Autodesk Inventor part; units mm, degrees
ref_plane "YZ Plane" through (0, 0, 0) normal (1, 0, 0) x (0, 1, 0)
ref_plane "XZ Plane" through (0, 0, 0) normal (0, 1, 0) x (-1, 0, 0)
ref_plane "XY Plane" through (0, 0, 0) normal (0, 0, 1) x (1, 0, 0)
sketch "Sketch1" plane through (0, 0, 0) normal (0, 1, 0) x (-1, 0, 0)
  circle A0 centre (0, 0) radius 46
  dimension "d2" = 92
extrude "Extrusion1" add sketch "Sketch1" along normal blind 28.5
chamfer "Chamfer1" distance 10 angle 45 2 edges at (46, 0, 0) (46, 28.5, 0)
sketch "Sketch2" plane through (0, 28.5, 0) normal (0, 1, 0) x (1, 0, 0)
  circle A0 centre (0, 0) radius 36
  circle A1 centre (0, 0) radius 7.5 construction
  point P0 (-0.3002, 0.0027)
  point P1 (9.3558, -1.447)
  point P2 (7.5, 0)
  point P3 (0, -7.5)
  point P4 (-7.5, 0)
  point P5 (0, 7.5)
  dimension "d13" = 15
hole "Hole1" at (7.5, 28.5, 0) at (0, 28.5, 7.5) at (-7.5, 28.5, 0) at (0, 28.5, -7.5) direction (0, -1, 0) diameter 2.459 depth 8.8 tip angle 118
sketch "Sketch3" plane through (0, 28.5, 0) normal (0, -1, 0) x (1, 0, 0)
  circle A0 centre (0, 0) radius 2.5
  dimension "d14" = 5
extrude "Extrusion2" add sketch "Sketch3" against normal blind 5
properties part number "EAGLE POWER 8308"
Design review of the part built by this model. Coordinates are the model's own, in mm. A direction names the side the tool comes from. Round coordinates to 2 decimals unless told otherwise and drop trailing zeros. Write each loop counter-clockwise with the first axis right and the second up, starting at its lowest first coordinate (ties: lowest second). Pieces come first, ordered by that corner, then holes.
Item 1: We need section B-B on y = 6.5. Write out the cut boundary in (x, z), and give its area (3 significant figures).
Item 2: For faces 4 (the flat face through (0, 33.5, 0)), 5 (the cylindrical face through (-0.369, 24.038, 8.673)), list the 3-axis set-ups (+Z, -Z, +X, -X, +Y, -Y) from which the entire face can be reached by the end or side of a thin tool; tool diameter is ignored.
Item 3: Clearance check with flat-ended pins moving along their axes: pin 1 Ø6 at (x, z) = (25.5, -16) entering from +Y; pin 2 Ø8 at (x, y) = (-21.5, 21) entering from +Z; pin 3 Ø10 at (y, z) = (29.5, 33) entering from -X; pin 4 Ø2 at (x, z) = (0, -7.5) entering from -Y. State where each tip first meets the part, or that it passes through.
Item 4: For probe 1 along X at (y, z) = (22, 0); probe 2 along X at (y, z) = (22.5, 0); probe 3 along Y at (x, z) = (-9.5, -18), list the stretches that pass through material, from the lowest coordinate up.
Item 5: The part is to be moulded in two halves that separate along Z. For faces 1 (the conical face through (0.064, 19.09, 7.704)), 2 (the cylindrical face through (-0.54, 30.96, -2.44)), 3 (the flat face through (1, 0, 1)), say which applies: +Z half, -Z half, draft (parallel to the pull), parting line (faces both ways), or undercut.
Item 6: We need section A-A on y = 27. Write out the cut boundary in (x, z).
Returned:
1. outline: circle Ø85 at (0, 0)
1. area: 5,670 mm2
2. face 4: +Z, -Z, +X, -X, +Y
2. face 5: +Y
3. pin 1: stops at y = 28.5
3. pin 2: stops at z = 42.17
3. pin 3: stops at x = -24.92
3. pin 4: stops at y = 0
4. probe 1: x = -42.5 to -8.73, -6.27 to 6.27, 8.73 to 42.5
4. probe 2: x = -42 to -8.73, -6.27 to 6.27, 8.73 to 42
4. probe 3: y = 0 to 28.5
5. face 1: undercut
5. face 2: parting line
5. face 3: draft
6. outline: circle Ø75 at (0, 0); hole circle Ø2.46 at (-7.5, 0); hole circle Ø2.46 at (0, -7.5); hole circle Ø2.46 at (0, 7.5); hole circle Ø2.46 at (7.5, 0)
